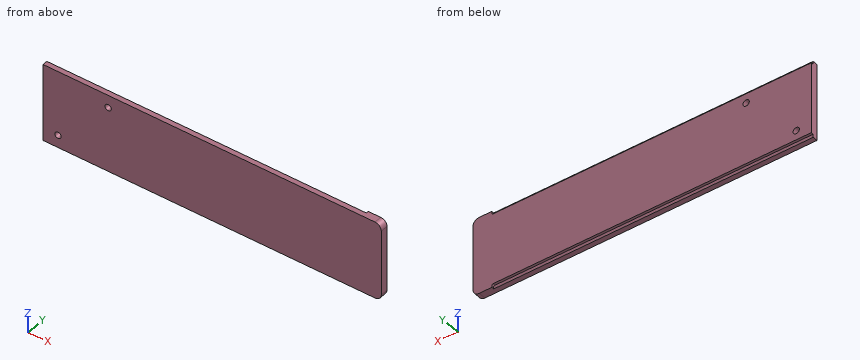
from build123d import *

# Parameters (mm, degrees)
SKETCH1_W           = 270
SKETCH1_H           = 62
BOSS_EXTRUDE1_DEPTH = 6
SKETCH2_W           = 255
SKETCH2_H           = 2.5
CUT_EXTRUDE1_DEPTH  = 2
FILLET1_R           = 1
SKETCH3_R           = 2.5
CUT_EXTRUDE2_DEPTH  = 7
FILLET2_R           = 5


with BuildPart() as part:
    # Sketch1 → Boss-Extrude1 (new body)
    with BuildSketch(Plane(origin=(0, 0, 0), x_dir=(1, 0, 0), z_dir=(0, 1, 0))):
        with Locations((135, 31)):
            Rectangle(SKETCH1_W, SKETCH1_H)
    extrude(amount=BOSS_EXTRUDE1_DEPTH)

    # Sketch2 → Cut-Extrude1 (cut)
    with BuildSketch(Plane(origin=(0, 6, 0), x_dir=(1, 0, 0), z_dir=(0, 1, 0))):
        with Locations((127.5, 60.75)):
            Rectangle(SKETCH2_W, SKETCH2_H)
        with Locations((127.5, 1.25)):
            Rectangle(SKETCH2_W, SKETCH2_H)
    extrude(amount=-CUT_EXTRUDE1_DEPTH, mode=Mode.SUBTRACT)

    # Fillet1
    fillet1_edges = [part.edges().sort_by_distance(p)[0] for p in [
        (255, 5, -59.5),
        (255, 5, -2.5),
    ]]
    fillet(fillet1_edges, radius=FILLET1_R)

    # Sketch3 → Cut-Extrude2 (cut, through all)
    with BuildSketch(Plane(origin=(0, 6, 0), x_dir=(1, 0, 0), z_dir=(0, 1, 0))):
        with Locations((12, 52)):
            Circle(SKETCH3_R)
        with Locations((52, 10)):
            Circle(SKETCH3_R)
    extrude(amount=-CUT_EXTRUDE2_DEPTH, mode=Mode.SUBTRACT)

    # Fillet2
    fillet2_edges = [part.edges().sort_by_distance(p)[0] for p in [
        (270, 3, -62),
        (270, 3, 0),
    ]]
    fillet(fillet2_edges, radius=FILLET2_R)


solid = part.part
Can you work these out from the model? Positions are in its coordinate system, mm. Coordinates: 2 decimals unless noted, no trailing zeros. Order: outer loops, then holes, each group sorted by start corner. A loop starts at its lowest first (then second) coordinate and runs counter-clockwise, first axis right, second up. Notation, with made-up numbers: (82.25, 24.25) -> (110.25, 24.25) arc R32 cw to (110.25, 55.25) -> close; hole circle Ø3 at (47.25, -8.5). An arc over 180 degrees is marked (long way). Use one line per item in the form item = value.
Q1. Imagine slicing it at B-B, the plane x = 52. List the corners of the cut face in (y, z) for me.
From the geometry:
outline = (0, -62) -> (4, -62) -> (4, -59.5) -> (6, -59.5) -> (6, -12.5) -> (0, -12.5) -> close; (0, -7.5) -> (6, -7.5) -> (6, -2.5) -> (4, -2.5) -> (4, 0) -> (0, 0) -> close
Q2. Will these pins go through, and if not, where does the flat tip stop? P1, Ø0.5, axis at y = 4.5, z = -1, coming from the -X side; P2, Ø1, axis at y = 2.5, z = -50, coming from the -X side; P3, Ø0.6, axis at x = 144, y = 5.5, coming from the -Z side; P4, Ø2, axis at x = 84.5, z = -0.5, coming from the +Y side.
From the geometry:
P1 = 255
P2 = 0
P3 = -59.5
P4 = 4
Q3. I need wall thicknesses on L1, parallel to X at y = 3, z = -52; L2, parallel to X at y = 4.95, z = -10.5; L3, parallel to Z at x = 12, y = 3.9. Which ranges of each line are inside material? Lowest first, please.
From the geometry:
L1 = 0 to 9.5, 14.5 to 270
L2 = 0 to 49.55, 54.45 to 270
L3 = -62 to -54.5, -49.5 to 0
Q4. Imagine slicing it at A-A, the plane z = -52. List the corners of the cut face in (x, y) for me.
From the geometry:
outline = (0, 0) -> (9.5, 0) -> (9.5, 6) -> (0, 6) -> close; (14.5, 0) -> (270, 0) -> (270, 6) -> (14.5, 6) -> close
Q5. Imagine slicing it at C-C, the plane x = 193.5. List the corners of the cut face in (y, z) for me, then the cut area to 3 significant figures.
From the geometry:
outline = (0, -62) -> (4, -62) -> (4, -59.5) -> (6, -59.5) -> (6, -2.5) -> (4, -2.5) -> (4, 0) -> (0, 0) -> close
area = 362 mm²
